Solid Edge part; units mm, degrees
sketch "Sketch1" plane through (0, 0, 0) normal (0, -1, 0) x (1, 0, 0)
  line L0 (-33.8082, 27.0293) -> (-33.8082, 15.6714)
  line L1 (-28.21, 15.6714) -> (-33.8082, 15.6714)
  line L2 (-16.9516, 22.1714) -> (-28.21, 15.6714)
  line L3 (-16.9516, 22.1714) -> (-13.3234, 22.1714)
  line L4 (-2.0651, 15.6714) -> (-13.3234, 22.1714)
  line L5 (-2.0651, 15.6714) -> (-2.0651, 9.6714)
  line L6 (-2.0651, 9.6714) -> (-43.4375, 9.6714)
  line L7 (-43.4375, 9.6714) -> (-43.4375, 27.0293)
  line L8 (-43.4375, 27.0293) -> (-33.8082, 27.0293)
extrude "ExtrudedProtrusion_1" add sketch "Sketch1" along normal blind 95
sketch "Sketch2" plane through (-22.7513, -47.5, 9.6714) normal (0, 0, -1) x (1, 0, 0)
  circle A0 centre (-15.8662, -31.4) radius 2.2
  circle A1 centre (-15.8662, 0) radius 2.2
  circle A2 centre (-15.8662, 35.8) radius 2.2
extrude "Cutout1" cut sketch "Sketch2" against normal blind 152.8035
sketch "Sketch3" plane through (-7.6943, -47.5, 18.9214) normal (0.5, 0, 0.866) x (0, 1, 0)
  circle A0 centre (41, 0) radius 2.2
  circle A1 centre (-41, 0) radius 2.2
extrude "ExtrudedCutout_2" cut sketch "Sketch3" against normal blind 455.9442
sketch "Sketch4" plane through (-22.5808, -47.5, 18.9214) normal (-0.5, 0, 0.866) x (0, -1, 0)
  circle A0 centre (32.2, 0) radius 2.2
  circle A1 centre (-32.6, 0) radius 2.2
extrude "ExtrudedCutout_3" cut sketch "Sketch4" against normal blind 76.0827
sketch "Sketch5" plane through (-2.0651, -47.5, 12.6714) normal (1, 0, 0) x (0, 1, 0)
  line L0 (-25.7, -3) -> (-25.7, 11)
  line L1 (-25.7, 11) -> (26.1, 11)
  line L2 (26.1, 11) -> (26.1, -3)
  line L3 (26.1, -3) -> (-25.7, -3)
extrude "ExtrudedCutout_4" cut sketch "Sketch5" against normal blind 31.7196
Geometry check sheet. Reference: the model listing, model coordinates, mm. A direction names the side the tool comes from. Coordinates: 2 decimals unless noted, no trailing zeros. Order: outer loops, then holes, each group sorted by start corner. A loop starts at its lowest first (then second) coordinate and runs counter-clockwise, first axis right, second up. Notation, with made-up numbers: M 79.5,-39.5 L 119.5,-39.5 A12 cw 119.5,-26.5 Z; hole C 57,33.5 d10. An arc over 180 degrees is marked long. One line per question, with ' | ' between items. Start each with the question number.
Item 1: Set-up check for faces 4 (the flat face through (-15, -84, 22.171)), 5 (the cylindrical face through (-12.53, -6.79, 14.91)), 6 (the flat face through (-33.785, -48, 13)), 7 (the flat face through (-22.5, -10.55, 18.97)): record each of +Z, -Z, +X, -X, +Y, -Y from which the full face is reachable in a straight line by a thin tool's end or side.
Item 2: Material ranges on L1, parallel to Y at x = -31.5, z = 14.5; L2, parallel to X at y = -16.1, z = 19.25; L3, parallel to X at y = -83.3, z = 14.5, recorded low to high. Write a range as [from, to].
Item 3: Cross-section at C-C on x = -27. Enter the section's corners in (y, z).
Item 4: Cross-section at D-D on z = 25.25. Enter the section's corners in (x, y).
Item 5: Gauge pin test, flat ends, axial feed: pin 1 (3 mm diameter, centred on x = -16, y = -79.5, fed in from +Z); pin 2 (3.5 mm diameter, centred on y = -66.5, z = 20, fed in from +X); pin 3 (2.5 mm diameter, centred on x = -38.62, y = -47.5, fed in from -Z). Record the tip position at first contact, or that the pin passes through.
Item 6: Cross-section at B-B on y = -16.1. Enter the section's corners in (x, z).
Item 7: Draft check along X on faces 1 (the cylindrical face through (-39.09, -45.35, 18.23)), 2 (the flat face through (-22, -95, 16)), 3 (the flat face through (-2.065, -84, 13)). Enter one of: pulls with the +X half, pulls with the -X half, needs draft (parallel to the pull), parting line crosses it, or undercut.
Findings:
1) face 4: +Z, +X, +Y, -Y | face 5: none | face 6: +Z, -Z, +X | face 7: +Z, +Y, -Y
2) L1: y = [-95, -73.2], [-21.4, 0] | L2: x = [-43.44, -40.82], [-36.42, -33.81], [-20.64, -8.26] | L3: x = [-43.44, -40.82], [-36.42, -2.07]
3) outline: M -95,9.67 L -73.2,9.67 L -73.2,16.37 L -95,16.37 Z; M -21.4,9.67 L 0,9.67 L 0,16.37 L -21.4,16.37 Z
4) outline: M -43.44,-95 L -33.81,-95 L -33.81,0 L -43.44,0 Z; hole C -38.62,-83.3 d4.4; hole C -38.62,-47.5 d4.4; hole C -38.62,-16.1 d4.4
5) pin 1: stops at z = 22.17 | pin 2: stops at x = -33.81 | pin 3: passes through
6) outline: M -43.44,9.67 L -40.82,9.67 L -40.82,27.03 L -43.44,27.03 Z; M -36.42,9.67 L -19.37,9.67 L -24.18,18 L -28.21,15.67 L -33.81,15.67 L -33.81,27.03 L -36.42,27.03 Z; M -20.98,19.84 L -15.11,9.67 L -2.07,9.67 L -2.07,15.67 L -13.32,22.17 L -16.95,22.17 Z
7) face 1: undercut | face 2: needs draft | face 3: pulls with the +X half
